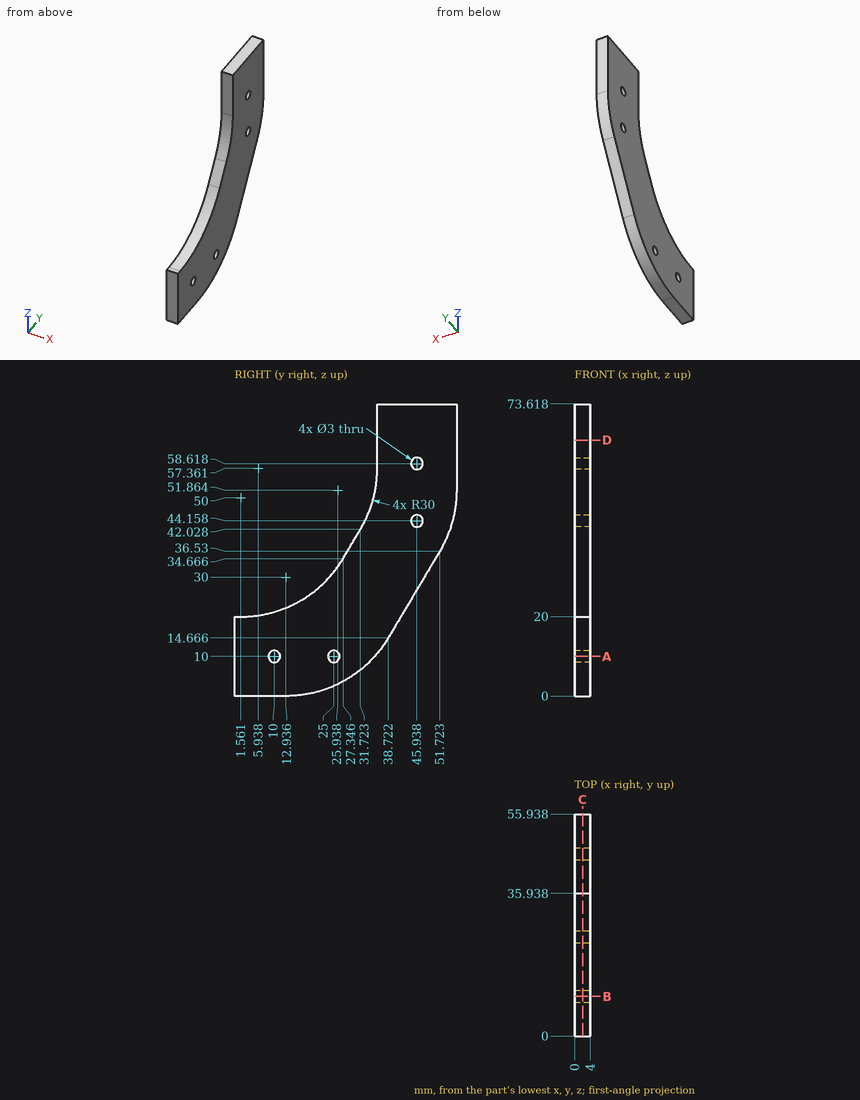
Study the drawing (mm; zero at the part's minimum x, y, z) and answer. Give positions to 0.01 mm unless a question says otherwise; leave off trailing zeros. Order: outer loops, then holes, each group sorted by start corner. A loop starts at its lowest first (then second) coordinate and runs counter-clockwise, first axis right, second up. Notation, with made-up numbers: (19, -11) - (71, -11) arc R26 ccw to (71, 15) - close; hole circle Ø7 at (-14.75, -40). An arc over 180 degrees is marked (long way). Answer in a Markdown table with one row per item. Add a question column.
Q1. The part is cut by section D-D (z = 64.5). Determine the outline of the cut face in (x, y), then the cut area to 3 significant figures.
Q2. Find the intervals of material crossed by line 1 along Y through (x, z) = (2.75, 10) (1 decimal); line 2 along Z through (x, y) = (3.3, 46) (1 decimal); line 3 along Y through (x, z) = (0.2, 64), in increasing order. Write a range as [from, to].
Q3. The part is cut by section A-A (z = 10). Determine the outline of the cut face in (x, y).
Q4. Given P1, Ø1.8, axis at y = 45.94, z = 58.62, coming from the -X side; P2, Ø4, axis at y = 50, z = 54.5, coming from the -X side; P3, Ø1, axis at x = 3.5, y = 7, coming from the +Z side; P4, Ø1.2, axis at x = 1, z = 69, coming from the -Y side, each flat-ended and moving along its own axis, determine where each tip first touches the part or whether it passes through.
Q5. The part is cut by section C-C (x = 2.05). Determine the outline of the cut face in (y, z) (1 decimal).
Q6. The part is cut by section B-B (y = 10). Determine the outline of the cut face in (x, z).
Determined:
| question | item | result |
|---|---|---|
| 1 | outline | (0, 35.94) - (4, 35.94) - (4, 55.94) - (0, 55.94) - close |
| 1 | area | 80.0 mm² |
| 2 | line 1 | y = [0, 8.5], [11.5, 23.5], [26.5, 35.3] |
| 2 | line 2 | z = [26.9, 42.7], [45.7, 57.1], [60.1, 73.6] |
| 2 | line 3 | y = [35.94, 55.94] |
| 3 | outline | (0, 0) - (4, 0) - (4, 8.5) - (0, 8.5) - close; (0, 11.5) - (4, 11.5) - (4, 23.5) - (0, 23.5) - close; (0, 26.5) - (4, 26.5) - (4, 35.3) - (0, 35.3) - close |
| 4 | P1 | passes through |
| 4 | P2 | stops at x = 0 |
| 4 | P3 | stops at z = 20.59 |
| 4 | P4 | stops at y = 35.94 |
| 5 | outline | (0, 0) - (12.9, 0) arc R30 ccw to (38.7, 14.7) - (51.7, 36.5) arc R30 ccw to (55.9, 51.9) - (55.9, 73.6) - (35.9, 73.6) - (35.9, 57.4) arc R30 cw to (31.7, 42) - (27.3, 34.7) arc R30 cw to (1.6, 20) - (0, 20) - close; hole circle Ø3 at (10, 10); hole circle Ø3 at (25, 10); hole circle Ø3 at (45.9, 44.2); hole circle Ø3 at (45.9, 58.6) |
| 6 | outline | (0, 0) - (4, 0) - (4, 8.5) - (0, 8.5) - close; (0, 11.5) - (4, 11.5) - (4, 21.21) - (0, 21.21) - close |
